Could you check a few things on this model? Use its own coordinates, in mm. A direction names the side the tool comes from. Give positions to 0.01 mm unless a question says otherwise; leave off trailing zeros. Loops run counter-clockwise (first coordinate to the right, second up) from the corner with the lowest first, then second, coordinate; pieces in that order, holes last. Notation, with made-up numbers: M -30,43 L 8,43 A19 cw 8,79 Z; hole C 22,18.5 d6. An arc over 180 degrees is marked long. Use a Markdown table: item, result. Add a question column.
1) Will these pins go through, and if not, where does the flat tip stop? pin 1 Ø1.2 at (x, y) = (0, 0.5) entering from -Z; pin 2 Ø1 at (y, z) = (-1.5, 9) entering from -X; pin 3 Ø1 at (y, z) = (0, 8) entering from +X.
2) Suppose I cut it at A-A on x = 0. List the corners of the cut face in (y, z) for me.
3) Suppose I cut it at B-B on z = 5.5. List the corners of the cut face in (x, y) for me, and give its area (3 significant figures).
4) If I drill on line 1 along Y through (x, z) = (0, 1.75); line 2 along Z through (x, y) = (-0.4, -1.55); line 3 along Y through (x, z) = (1, 3.75), over which ranges is the centre line in solid material (lowest first)? Write a range as [from, to].
5) Which directions (+Z, -Z, +X, -X, +Y, -Y) give clear straight access to the entire face, cutting with the end or side of a thin tool? Please do faces 5 (the cylindrical face through (-1.5, -0.07, 7.81)), 6 (the flat face through (0, 0, 11)), 7 (the cylindrical face through (0.748, -0.976, 2.282)).
6) We'd pull the mould along X, two halves only. Please class faces 1 (the flat face through (2.026, 1.191, 2.465)), 2 (the flat face through (-2.045, 1.159, 2.465)), 3 (the flat face through (0, 2, 5)), 4 (the flat face through (0, 0, 4.5)): +X half, -X half, draft (parallel to the pull), parting line (faces both ways), or undercut.
Autodesk Inventor part; units mm, degrees
ref_plane "YZ Plane" through (0, 0, 0) normal (1, 0, 0) x (0, 1, 0)
ref_plane "XZ Plane" through (0, 0, 0) normal (0, 1, 0) x (-1, 0, 0)
ref_plane "XY Plane" through (0, 0, 0) normal (0, 0, 1) x (1, 0, 0)
sketch "Sketch1" plane through (0, 0, 0) normal (0, 0, 1) x (1, 0, 0)
  line L0 (2.7135, 0) -> (1.3568, -2.35)
  line L1 (1.3568, -2.35) -> (-1.3568, -2.35)
  line L2 (-1.3568, -2.35) -> (-2.7135, 0)
  line L3 (-2.7135, 0) -> (-1.3568, 2.35)
  line L4 (-1.3568, 2.35) -> (1.3568, 2.35)
  line L5 (1.3568, 2.35) -> (2.7135, 0)
  point P0 (0, 0)
  point P1 (0, 0)
  dimension "d0" = 4.7
extrude "Extrusion1" add sketch "Sketch1" along normal blind 5
sketch "Sketch2" plane through (0, 0, 5) normal (0, 0, 1) x (1, 0, 0)
  circle A0 centre (0, 0) radius 1.5
  dimension "d3" = 3
extrude "Extrusion2" add sketch "Sketch2" along normal blind 6
thread "Thread1"
chamfer "Chamfer1" distance 0.3 angle 45 1 edges at (-1.5, 0, 11)
sketch "Sketch3" plane through (0, 0, 0) normal (0, 0, -1) x (-1, 0, 0)
  point P0 (0, 0)
  point P1 (0, 0)
hole "Hole1" at (0, 0, 0) direction (0, 0, 1) diameter 2.459 depth 4.5
properties part number "5mm M3 Brass Standoff"
Answer block:
| question | item | result |
|---|---|---|
| 1 | pin 1 | stops at z = 4.5 |
| 1 | pin 2 | stops at x = -1.12 |
| 1 | pin 3 | stops at x = 1.5 |
| 2 | outline | M -2.35,0 L -1.23,0 L -1.23,4.5 L 1.23,4.5 L 1.23,0 L 2.35,0 L 2.35,5 L 1.5,5 L 1.5,10.7 L 1.2,11 L -1.2,11 L -1.5,10.7 L -1.5,5 L -2.35,5 Z |
| 3 | outline | C 0,0 d3 |
| 3 | area | 7.07 mm^2 |
| 4 | line 1 | y = [-2.35, -1.23], [1.23, 2.35] |
| 4 | line 2 | z = [0, 5] |
| 4 | line 3 | y = [-2.35, -0.72], [0.72, 2.35] |
| 5 | face 5 | +Z |
| 5 | face 6 | +Z, +X, -X, +Y, -Y |
| 5 | face 7 | -Z |
| 6 | face 1 | +X half |
| 6 | face 2 | -X half |
| 6 | face 3 | draft |
| 6 | face 4 | undercut |
